from build123d import *

# Parameters (mm, degrees)
PAD008_DEPTH  = 22
PAD008_TAPER  = 1.5
SKETCH016_R   = 2.5
HOLE004_DEPTH = 69.506788
SKETCH017_R   = 5
PAD009_DEPTH  = 15
HOLE005_DEPTH = 25


with BuildPart() as part:
    # Sketch015 → Pad008 (new body)
    with BuildSketch(Plane.XY):
        Polygon((10, 0), (5, 8.660254), (-5, 8.660254), (-10, 0), (-5, -8.660254), (5, -8.660254), align=None)
    extrude(amount=PAD008_DEPTH, taper=PAD008_TAPER)

    # Sketch016 → Hole004 (cut)
    with BuildSketch(Plane.XY):
        Circle(SKETCH016_R)
    extrude(amount=HOLE004_DEPTH, mode=Mode.SUBTRACT)

    # Sketch017 → Pad009 (join)
    with BuildSketch(Plane.XY):
        Circle(SKETCH017_R)
    extrude(amount=-PAD009_DEPTH)

    # Sketch016 → Hole005 (cut)
    with BuildSketch(Plane.XY):
        Circle(SKETCH016_R)
    extrude(amount=-HOLE005_DEPTH, mode=Mode.SUBTRACT)


with BuildPart() as part_1:
    # Body007 placement: moved
    add(part.part.moved(Location((0, 31.5, 21.4))))


solid = part_1.part
Verification items for the finished model (mm, model axes). A direction names the side the tool comes from. Give positions to 0.01 mm unless a question says otherwise; leave off trailing zeros. Write each loop counter-clockwise with the first axis right and the second up, starting at its lowest first coordinate (ties: lowest second). Pieces come first, ordered by that corner, then holes. Notation, with made-up numbers: M 39.5,51.5 L 82.5,51.5 A9 ccw 82.5,61.5 Z; hole C 74,-31.5 d11. An arc over 180 degrees is marked long. Put each result on its own line as item: value. Start each with the question number.
1. Set-up check for faces 1 (the face through (1.9, 33.4, 43.4)), 2 (the face through (4, 35, 21.4)): record each of +Z, -Z, +X, -X, +Y, -Y from which the full face is reachable in a straight line by a thin tool's end or side.
2. Scan lines: line 1 along X through (y, z) = (31.5, 23); line 2 along Z through (x, y) = (-0.25, 23.5); line 3 along Y through (x, z) = (0, 24.5). Record each from-to range of solid material in increasing order. Write a range as [from, to].
3. Section check B-B (z = 32). Record the cut outline in (x, y), and give its area (3 significant figures).
4. Section check D-D (y = 27). Record the cut outline in (x, z), and give its area (3 significant figures).
5. Section check A-A (x = 0). Record the cut outline in (y, z).
6. Draft check along X on faces 3 (the face through (1, 34, 6.4)), 4 (the face through (1.34, 33.61, 25.16)), 5 (the face through (-1.08, 26.62, 14)). Enter one of: +X half, -X half, draft (parallel to the pull), parting line (faces both ways), or undercut.
7. Go/stop test with flat-tipped pins: pin 1 Ø1 at (x, z) = (-3, 22.5) entering from -Y; pin 2 Ø4 at (y, z) = (28, 11) entering from +X; pin 3 Ø10 at (x, z) = (-3.5, 33.5) entering from +Y. Record where each tip stops, or that it passes through.
8. Section check C-C (y = 32.25). Record the cut outline in (x, z), and give its area (3 significant figures).
Answer list:
1. face 1: +Z, +X, -X, +Y, -Y
1. face 2: -Z
2. line 1: [-9.95, -2.5], [2.5, 9.95]
2. line 2: [21.4, 43.4]
2. line 3: [22.92, 29], [34, 40.08]
3. outline: M -9.68,31.5 L -4.84,23.12 L 4.84,23.12 L 9.68,31.5 L 4.84,39.88 L -4.84,39.88 Z; hole C 0,31.5 d5
3. area: 224 mm2
4. outline: M -7.4,21.4 L -2.18,21.4 L -2.18,6.4 L 2.18,6.4 L 2.18,21.4 L 7.4,21.4 L 6.74,43.4 L -6.74,43.4 Z
4. area: 376 mm2
5. outline: M 22.84,21.4 L 26.5,21.4 L 26.5,6.4 L 29,6.4 L 29,43.4 L 23.42,43.4 Z; M 34,6.4 L 36.5,6.4 L 36.5,21.4 L 40.16,21.4 L 39.58,43.4 L 34,43.4 Z
6. face 3: draft
6. face 4: undercut
6. face 5: parting line
7. pin 1: y = 22.86
7. pin 2: x = 4.77
7. pin 3: y = 39.97
8. outline: M -9.57,21.4 L -4.94,21.4 L -4.94,6.4 L -2.38,6.4 L -2.38,43.4 L -8.9,43.4 Z; M 2.38,6.4 L 4.94,6.4 L 4.94,21.4 L 9.57,21.4 L 8.9,43.4 L 2.38,43.4 Z
8. area: 378 mm2
